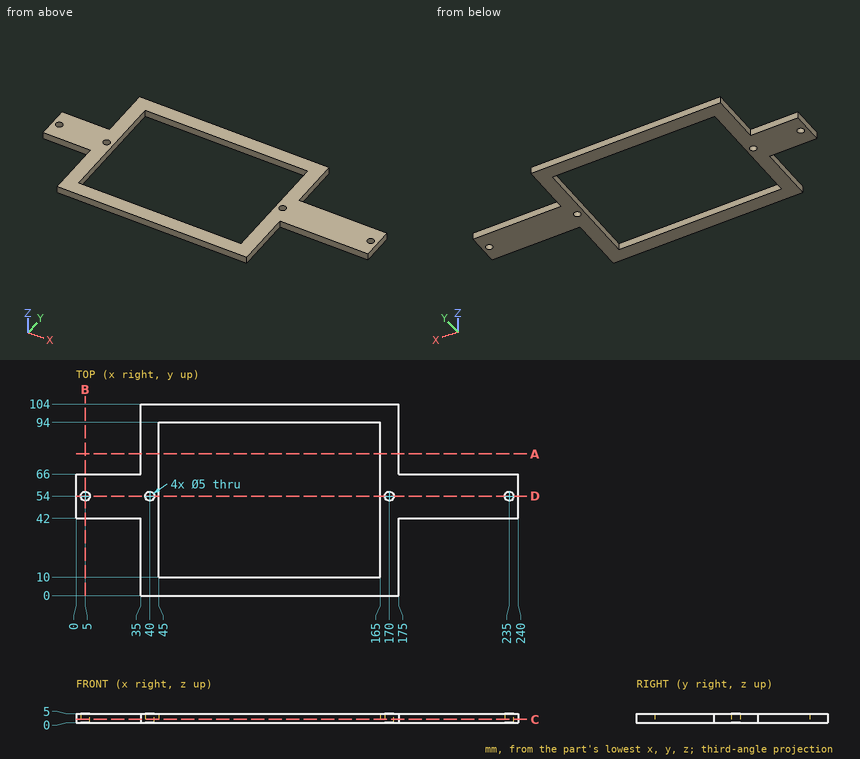
Input: dimensioned drawing with shaded views. Units: mm. Origin: part minimum x, y, z. Round coordinates to 2 decimals unless told otherwise and drop trailing zeros. Loops run counter-clockwise (first coordinate to the right, second up) from the corner with the lowest first, then second, coordinate; pieces in that order, holes last. Notation, with made-up numbers: (43, 88) -> (56, 88) arc R20 ccw to (56, 123) -> close; hole circle Ø6 at (-9, -24.5). An arc over 180 degrees is marked (long way). Use one line per item in the form item = value. Start each with the question number.
1) Section B-B on x = 5. Output: boundary loops of the cut face in (y, z), then the cut area to 3 significant figures.
2) Line query: L1, parallel to X at y = 54, z = 2.8; L2, parallel to Y at x = 40, z = 1.1; L3, parallel to Y at x = 5, z = 4. Output: solid intervals per line, ascending.
3) Section C-C on z = 1.9. Output: boundary loops of the cut face in (x, y).
4) Section D-D on y = 54. Output: boundary loops of the cut face in (x, z), then the cut area to 3 significant figures.
5) Section A-A on y = 77. Output: boundary loops of the cut face in (x, z), then the cut area to 3 significant figures.
6) First-contact query: P1, Ø1.5, axis at x = 196.5, z = 3.5, coming from the +Y side; P2, Ø1.5, axis at x = 11.5, z = 2, coming from the -Y side; P3, Ø3, axis at y = 38.5, z = 4.5, coming from the +X side; P4, Ø6.5, axis at x = 5, y = 54, coming from the +Z side. Flat tips, straight axial feed; report the tip coordinate or a pass-through.
Response:
q1.outline = (42, 0) -> (51.5, 0) -> (51.5, 5) -> (42, 5) -> close; (56.5, 0) -> (66, 0) -> (66, 5) -> (56.5, 5) -> close
q1.area = 95.0 mm^2
q2.L1 = 0 to 2.5, 7.5 to 37.5, 42.5 to 45, 165 to 167.5, 172.5 to 232.5, 237.5 to 240
q2.L2 = 0 to 51.5, 56.5 to 104
q2.L3 = 42 to 51.5, 56.5 to 66
q3.outline = (0, 42) -> (35, 42) -> (35, 0) -> (175, 0) -> (175, 42) -> (240, 42) -> (240, 66) -> (175, 66) -> (175, 104) -> (35, 104) -> (35, 66) -> (0, 66) -> close; hole circle Ø5 at (5, 54); hole circle Ø5 at (40, 54); hole (45, 10) -> (165, 10) -> (165, 94) -> (45, 94) -> close; hole circle Ø5 at (170, 54); hole circle Ø5 at (235, 54)
q4.outline = (0, 0) -> (2.5, 0) -> (2.5, 5) -> (0, 5) -> close; (7.5, 0) -> (37.5, 0) -> (37.5, 5) -> (7.5, 5) -> close; (42.5, 0) -> (45, 0) -> (45, 5) -> (42.5, 5) -> close; (165, 0) -> (167.5, 0) -> (167.5, 5) -> (165, 5) -> close; (172.5, 0) -> (232.5, 0) -> (232.5, 5) -> (172.5, 5) -> close; (237.5, 0) -> (240, 0) -> (240, 5) -> (237.5, 5) -> close
q4.area = 500 mm^2
q5.outline = (35, 0) -> (45, 0) -> (45, 5) -> (35, 5) -> close; (165, 0) -> (175, 0) -> (175, 5) -> (165, 5) -> close
q5.area = 100 mm^2
q6.P1 = 66
q6.P2 = 42
q6.P3 = 175
q6.P4 = 5
